Autodesk Inventor part; units mm, degrees
ref_plane "to_collar_XY" through (-1, 0, 0) normal (-1, 0, 0) x (0, -0.7071068, -0.7071068)
ref_plane "to_collar_YZ" through (-1, 0, 0) normal (0, -0.7071068, -0.7071068) x (0, -0.7071068, 0.7071068)
ref_plane "to_collar_ZX" through (-1, 0, 0) normal (0, -0.7071068, 0.7071068) x (-1, 0, 0)
sketch "Sketch_1" plane through (0, 0, 0) normal (1, 0, 0) x (0, 0, -1)
  line L0 (-8, 6) -> (-8, -6)
  arc A0 (-8, -6) -> (-6, -8) centre (0, 0) ccw
  line L1 (-6, -8) -> (6, -8)
  arc A1 (6, -8) -> (8, -6) centre (0, 0) ccw
  line L2 (8, -6) -> (8, 6)
  arc A2 (8, 6) -> (6, 8) centre (0, 0) ccw
  line L3 (6, 8) -> (-6, 8)
  arc A3 (-6, 8) -> (-8, 6) centre (0, 0) ccw
extrude "Extrusion1" add sketch "Sketch_1" along normal blind 7
sketch "Sketch_2" plane through (0, 0, 0) normal (0, 0, 1) x (1, 0, 0)
  line L0 (0, 0) -> (-1, 0)
  line L1 (-1, 0) -> (-1, 7.5)
  line L2 (-1, 7.5) -> (0, 7.5)
  line L3 (0, 7.5) -> (0, 0)
  line L4 (0, 0) -> (-1, 0)
revolve "Revolution1" add sketch "Sketch_2" angle 360 about axis through (0, 0, 0) along (1, 0, 0)
sketch "Sketch_3" plane through (0, 0, 0) normal (0, 0, 1) x (1, 0, 0)
  line L0 (7, 0) -> (-1, 0)
  line L1 (-1, 0) -> (-1, 5)
  line L2 (-1, 5) -> (-0.4585, 4.4585)
  line L3 (-0.4585, 4.4585) -> (6.4585, 4.4585)
  line L4 (6.4585, 4.4585) -> (7, 5)
  line L5 (7, 5) -> (7, 0)
  line L6 (7, 0) -> (-1, 0)
revolve "Revolution2" cut sketch "Sketch_3" angle 360 about axis through (7, 0, 0) along (1, 0, 0)
thread "Thread1"
sketch "Sketch_4" plane through (4.5, 0, 0) normal (1, 0, 0) x (0, 0, -1)
  line L0 (0, 0) -> (7.0711, 7.0711)
  line L1 (7.0711, 7.0711) -> (8.1317, 6.0104)
  line L2 (8.1317, 6.0104) -> (7.7492, 6.0104)
  line L3 (7.7492, 6.0104) -> (0.8694, -0.8694)
  line L4 (0.8694, -0.8694) -> (0, 0)
  line L5 (0, 0) -> (7.0711, 7.0711)
revolve "Revolution3" cut sketch "Sketch_4" angle 360 about axis through (4.5, 0, 0) along (0, -0.7071068, 0.7071068)
thread "Thread2"
ref_plane "to_collar_XY" through (-1, 0, 0) normal (-1, 0, 0) x (0, -0.7071068, -0.7071068)
ref_plane "to_collar_YZ" through (-1, 0, 0) normal (0, -0.7071068, -0.7071068) x (0, -0.7071068, 0.7071068)
ref_plane "to_collar_ZX" through (-1, 0, 0) normal (0, -0.7071068, 0.7071068) x (-1, 0, 0)
properties part number "C-TFK10_n"
Design review of the part built by this model. Coordinates are the model's own, in mm. A direction names the side the tool comes from. Round coordinates to 2 decimals unless told otherwise and drop trailing zeros. Write each loop counter-clockwise with the first axis right and the second up, starting at its lowest first coordinate (ties: lowest second). Pieces come first, ordered by that corner, then holes.
Item 1: We need section B-B on x = 2.5. Write out the cut boundary in (y, z).
Item 2: For probe 1 along Z at (x, y) = (2.5, 0); probe 2 along X at (y, z) = (-6.75, 4); probe 3 along X at (y, z) = (7.25, -6.75), list the stretches that pass through material, from the lowest coordinate up.
Item 3: The part is to be moulded in two halves that separate along Z. For faces 1 (the cylindrical face through (3.05, -3.54, -2.71)), 2 (the cylindrical face through (-0.493, -7.493, 0.33)), 3 (the flat face through (7, 4, 4)), say which applies: +Z half, -Z half, draft (parallel to the pull), parting line (faces both ways), or undercut.
Item 4: For faces 4 (the flat face through (0, -6, 5)), 5 (the cylindrical face through (3.451, -7.057, -7.085)), list the 3-axis set-ups (+Z, -Z, +X, -X, +Y, -Y) from which the entire face can be reached by the end or side of a thin tool; tool diameter is ignored.
Item 5: We need section D-D on z = 7.25. Write out the cut boundary in (x, y).
Item 6: We need section A-A on z = 0. Write out the cut boundary in (x, y).
Returned:
1. outline: (-8, -6) arc R10 ccw to (-6, -8) - (6, -8) arc R10 ccw to (8, -6) - (8, 6) arc R10 ccw to (6, 8) - (-6, 8) arc R10 ccw to (-8, 6) - close; hole circle Ø8.92 at (0, 0)
2. probe 1: z = -8 to -4.46, 4.46 to 8
2. probe 2: x = 0 to 7
2. probe 3: x = 0 to 3.15, 5.85 to 7
3. face 1: undercut
3. face 2: parting line
3. face 3: draft
4. face 4: -X
4. face 5: -Z, +X, -X, -Y
5. outline: (-1, -1.92) - (0, -1.92) - (0, -6.89) - (7, -6.89) - (7, 6.89) - (0, 6.89) - (0, 1.92) - (-1, 1.92) - close
6. outline: (-1, -7.5) - (0, -7.5) - (0, -8) - (7, -8) - (7, -5) - (6.46, -4.46) - (-0.46, -4.46) - (-1, -5) - close; (-1, 5) - (-0.46, 4.46) - (6.46, 4.46) - (7, 5) - (7, 8) - (0, 8) - (0, 7.5) - (-1, 7.5) - close
